Geometry check sheet. Reference: the model listing, model coordinates, mm. Round coordinates to 2 decimals unless told otherwise and drop trailing zeros. Write each loop counter-clockwise with the first axis right and the second up, starting at its lowest first coordinate (ties: lowest second). Pieces come first, ordered by that corner, then holes. Notation, with made-up numbers: (75, 8.5) - (127, 8.5) arc R17 cw to (127, 28.5) - close; hole circle Ø2 at (29.25, -3). An arc over 180 degrees is marked (long way). Return JSON: item names as keys, results as strings.
Autodesk Fusion 360 part; units mm, degrees
sketch "Sketch1" plane through (0, 0, 0) normal (0, 0, 1) x (1, 0, 0)
  line L0 (0, 0) -> (-50, 0)
  line L1 (-50, 0) -> (-50, 50)
  line L2 (-50, 50) -> (0, 50)
  line L3 (0, 50) -> (0, 0)
  circle A0 centre (-25, 25) radius 21
  dimension "d1" = 42
extrude "Extrude1" add sketch "Sketch1" along normal blind 4.78
(1) Section check C-C, the plane z = 1.75. Enter the section's corners in (x, y).
Response values:
{"outline": "(-50, 0) - (0, 0) - (0, 50) - (-50, 50) - close; hole circle Ø42 at (-25, 25)"}
(2) Section check B-B, the plane x = -25. Enter the section's corners in (y, z).
Response values:
{"outline": "(0, 0) - (4, 0) - (4, 4.78) - (0, 4.78) - close; (46, 0) - (50, 0) - (50, 4.78) - (46, 4.78) - close"}
(3) Release check for a two-part mould opening along X. For faces 1 (the face through (-25, 0, 2)), 2 (the face through (-5.6, 33.04, 2.36)), 3 (the face through (-50, 25, 2)) record: pulls with the +X half, pulls with the -X half, needs draft (parallel to the pull), parting line crosses it, or undercut.
Response values:
{"face 1": "needs draft", "face 2": "undercut", "face 3": "pulls with the -X half"}
(4) Section check A-A, the plane y = 25. Enter the section's corners in (x, z).
Response values:
{"outline": "(-50, 0) - (-46, 0) - (-46, 4.78) - (-50, 4.78) - close; (-4, 0) - (0, 0) - (0, 4.78) - (-4, 4.78) - close"}
(5) Material ranges on line 1 along Y through (x, z) = (-25, 1.65); line 2 along Y through (x, z) = (-43, 1.35); line 3 along X through (y, z) = (40, 2.9), recorded low to high. Write a range as [from, to].
Response values:
{"line 1": "y = [0, 4], [46, 50]", "line 2": "y = [0, 14.18], [35.82, 50]", "line 3": "x = [-50, -39.7], [-10.3, 0]"}
